Source: CAD feature listing. Evaluate the final solid. Frame: model axes, mm. Give positions to 0.01 mm unless a question says otherwise; leave off trailing zeros. Write each loop counter-clockwise with the first axis right and the second up, starting at its lowest first coordinate (ties: lowest second). Pieces come first, ordered by that corner, then holes. Notation, with made-up numbers: (34, 23.25) -> (79, 23.25) arc R22 cw to (79, 54.25) -> close; hole circle Ø10 at (-8, 27.5). An arc over 180 degrees is marked (long way). Use one line per item in the form item = value. Start each with the question number.
(1) Draft query along Z for faces 1 (the face through (-12.09, -0.03, 14.01)), 2 (the face through (0, 2, 0)), 3 (the face through (0, 0, 18.25)). Return one class per face: pulls with the +Z half, pulls with the -Z half, needs draft (parallel to the pull), parting line crosses it, or undercut.
(2) Cut plane A-A, the plane z = -15.25. Output: boundary loops of the cut face in (x, y), and give its area (3 significant figures).
(3) Material intervals for line 1 along Z through (x, y) = (12.25, 0.45); line 2 along X through (y, z) = (0.6, -15.25); line 3 along X through (y, z) = (0.6, 16), sorted ascending. Write a range as from..to.
(4) Cut plane B-B, the plane y = 0.7. Output: boundary loops of the cut face in (x, z).
(5) Cut plane C-C, the plane x = 12.25. Output: boundary loops of the cut face in (y, z).
(6) First-contact query: P1, Ø3, axis at x = -12.25, z = -15.25, coming from the +Y side. Flat tip, straight axial feed; report the tip coordinate or a pass-through.
from build123d import *

# Parameters (mm, degrees)
SKETCH1_W             = 24.5
SKETCH1_H             = 24.5
BOSS_EXTRUDE1_DEPTH   = 2
SKETCH2_W             = 30.5
SKETCH2_H             = 36.5
SKETCH2_W_2           = 24.5
SKETCH2_H_2           = 24.5
BOSS_EXTRUDE2_DEPTH   = 4
M3X0_5_TAPPED_HOLE1_D = 2.5


with BuildPart() as part:
    # Sketch1 → Boss-Extrude1 (new body, symmetric)
    with BuildSketch(Plane(origin=(0, 0, 0), x_dir=(1, 0, 0), z_dir=(0, 1, 0))):
        Rectangle(SKETCH1_W, SKETCH1_H)
    extrude(amount=BOSS_EXTRUDE1_DEPTH, both=True)

    # Sketch2 → Boss-Extrude2 (add)
    with BuildSketch(Plane(origin=(0, 2, 0), x_dir=(1, 0, 0), z_dir=(0, 1, 0))):
        Rectangle(SKETCH2_W, SKETCH2_H)
        Rectangle(SKETCH2_W_2, SKETCH2_H_2, mode=Mode.SUBTRACT)
    extrude(amount=-BOSS_EXTRUDE2_DEPTH)

    # M3x0.5 Tapped Hole1 (through all)
    with Locations(Plane(origin=(0, 2, 0), x_dir=(1, 0, 0), z_dir=(0, 1, 0))):
        with Locations((-12.25, 15.25), (12.25, 15.25), (-12.25, -15.25), (12.25, -15.25)):
            Hole(M3X0_5_TAPPED_HOLE1_D / 2)


solid = part.part
Geometry says:
q1.face_1 = undercut
q1.face_2 = needs draft
q1.face_3 = pulls with the +Z half
q2.outline = (-15.25, -2) -> (-13.5, -2) -> (-13.5, 2) -> (-15.25, 2) -> close; (-11, -2) -> (11, -2) -> (11, 2) -> (-11, 2) -> close; (13.5, -2) -> (15.25, -2) -> (15.25, 2) -> (13.5, 2) -> close
q2.area = 102 mm^2
q3.line_1 = -18.25..-16.5, -14..14, 16.5..18.25
q3.line_2 = -15.25..-13.5, -11..11, 13.5..15.25
q3.line_3 = -15.25..-13.25, -11.25..11.25, 13.25..15.25
q4.outline = (-15.25, -18.25) -> (15.25, -18.25) -> (15.25, 18.25) -> (-15.25, 18.25) -> close; hole circle Ø2.5 at (-12.25, -15.25); hole circle Ø2.5 at (-12.25, 15.25); hole circle Ø2.5 at (12.25, -15.25); hole circle Ø2.5 at (12.25, 15.25)
q5.outline = (-2, -18.25) -> (2, -18.25) -> (2, -16.5) -> (-2, -16.5) -> close; (-2, -14) -> (2, -14) -> (2, 14) -> (-2, 14) -> close; (-2, 16.5) -> (2, 16.5) -> (2, 18.25) -> (-2, 18.25) -> close
q6.P1 = 2
